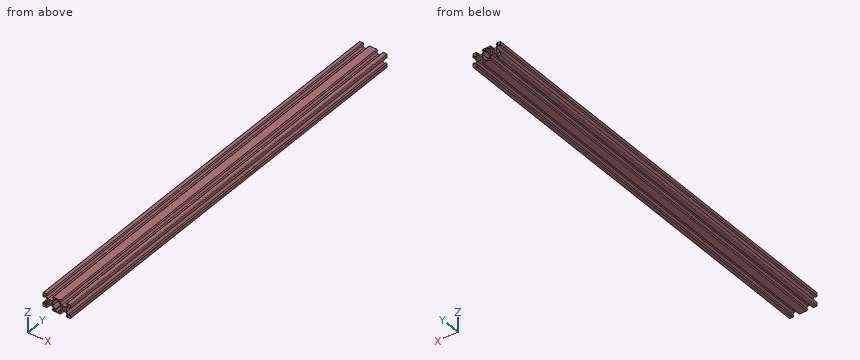
Autodesk Inventor part; units mm, degrees
ref_plane "YZ Plane" through (0, 0, 0) normal (1, 0, 0) x (0, 1, 0)
ref_plane "XZ Plane" through (0, 0, 0) normal (0, 1, 0) x (-1, 0, 0)
ref_plane "XY Plane" through (0, 0, 0) normal (0, 0, 1) x (1, 0, 0)
sketch "Sketch1" plane through (0, 0, 0) normal (0, 1, 0) x (-1, 0, 0)
  line L0 (3.9, -2.8393) -> (3.9, 2.8393)
  line L1 (2.8393, 3.9) -> (-2.8393, 3.9)
  line L2 (-2.8393, -3.9) -> (2.8393, -3.9)
  line L3 (8.5707, 3.2957) -> (10, 4.725)
  line L4 (8.5707, -3.2957) -> (10, -4.725)
  line L5 (8.4, 3.3664) -> (8.4, 6)
  line L6 (8.4, 6) -> (7.0607, 6)
  line L7 (10, 9) -> (10, 4.725)
  line L8 (10, -4.725) -> (10, -9)
  line L9 (3.9, 2.8393) -> (7.0607, 6)
  line L10 (3.2957, 8.5707) -> (4.725, 10)
  line L11 (3.3664, 8.4) -> (6, 8.4)
  line L12 (6, 8.4) -> (6, 7.0607)
  line L13 (2.8393, 3.9) -> (6, 7.0607)
  line L14 (8.4, -3.3664) -> (8.4, -6)
  line L15 (8.4, -6) -> (7.0607, -6)
  line L16 (3.9, -2.8393) -> (7.0607, -6)
  line L17 (3.2957, -8.5707) -> (4.725, -10)
  line L18 (3.3664, -8.4) -> (6, -8.4)
  line L19 (6, -8.4) -> (6, -7.0607)
  line L20 (2.8393, -3.9) -> (6, -7.0607)
  line L21 (-3.9, -2.8393) -> (-3.9, 2.8393)
  line L22 (-3.9, 2.8393) -> (-7.0607, 6)
  line L23 (-6, 8.4) -> (-6, 7.0607)
  line L24 (-2.8393, 3.9) -> (-6, 7.0607)
  line L25 (-3.9, -2.8393) -> (-7.0607, -6)
  line L26 (-2.8393, -3.9) -> (-6, -7.0607)
  line L27 (-6, -8.4) -> (-6, -7.0607)
  line L28 (-3.3664, -8.4) -> (-6, -8.4)
  line L29 (-3.2957, -8.5707) -> (-4.725, -10)
  line L30 (4.725, 10) -> (9, 10)
  line L31 (9, -10) -> (4.725, -10)
  circle A0 centre (0, 0) radius 2.1
  arc A1 (10, 9) -> (9, 10) centre (9, 9) ccw
  arc A2 (9, -10) -> (10, -9) centre (9, -9) ccw
  arc A3 (8.4, 3.3664) -> (8.5707, 3.2957) centre (8.5, 3.3664) ccw
  arc A4 (3.2957, 8.5707) -> (3.3664, 8.4) centre (3.3664, 8.5) ccw
  arc A5 (8.5707, -3.2957) -> (8.4, -3.3664) centre (8.5, -3.3664) ccw
  arc A6 (3.3664, -8.4) -> (3.2957, -8.5707) centre (3.3664, -8.5) ccw
  arc A7 (-3.2957, -8.5707) -> (-3.3664, -8.4) centre (-3.3664, -8.5) ccw
  line L32 (-23.9, -2.8393) -> (-23.9, 2.8393)
  line L33 (-22.8393, 3.9) -> (-17.1607, 3.9)
  line L34 (-17.1607, -3.9) -> (-22.8393, -3.9)
  line L35 (-28.5707, 3.2957) -> (-30, 4.725)
  line L36 (-28.5707, -3.2957) -> (-30, -4.725)
  line L37 (-28.4, 3.3664) -> (-28.4, 6)
  line L38 (-28.4, 6) -> (-27.0607, 6)
  line L39 (-30, 9) -> (-30, 4.725)
  line L40 (-30, -4.725) -> (-30, -9)
  line L41 (-23.9, 2.8393) -> (-27.0607, 6)
  line L42 (-23.2957, 8.5707) -> (-24.725, 10)
  line L43 (-23.3664, 8.4) -> (-26, 8.4)
  line L44 (-26, 8.4) -> (-26, 7.0607)
  line L45 (-22.8393, 3.9) -> (-26, 7.0607)
  line L46 (-23.9, 0) -> (-28.4, 0)
  line L47 (-23.9, -2.8393) -> (-27.0607, -6)
  line L48 (-28.4, -6) -> (-27.0607, -6)
  line L49 (-28.4, -3.3664) -> (-28.4, -6)
  line L50 (-22.8393, -3.9) -> (-26, -7.0607)
  line L51 (-26, -8.4) -> (-26, -7.0607)
  line L52 (-23.3664, -8.4) -> (-26, -8.4)
  line L53 (-23.2957, -8.5707) -> (-24.725, -10)
  line L54 (-16.1, -2.8393) -> (-12.9393, -6)
  line L55 (-17.1607, -3.9) -> (-14, -7.0607)
  line L56 (-16.6336, -8.4) -> (-14, -8.4)
  line L57 (-16.1, -2.8393) -> (-16.1, 2.8393)
  line L58 (-16.1, 2.8393) -> (-12.9393, 6)
  line L59 (-17.1607, 3.9) -> (-14, 7.0607)
  line L60 (-14, 8.4) -> (-14, 7.0607)
  line L61 (-14, -8.4) -> (-14, -7.0607)
  line L62 (-16.7043, -8.5707) -> (-15.275, -10)
  line L63 (-24.725, 10) -> (-29, 10)
  line L64 (-29, -10) -> (-24.725, -10)
  circle A8 centre (-20, 0) radius 2.1
  arc A9 (-29, 10) -> (-30, 9) centre (-29, 9) ccw
  arc A10 (-30, -9) -> (-29, -10) centre (-29, -9) ccw
  arc A11 (-28.5707, 3.2957) -> (-28.4, 3.3664) centre (-28.5, 3.3664) ccw
  arc A12 (-23.3664, 8.4) -> (-23.2957, 8.5707) centre (-23.3664, 8.5) ccw
  arc A13 (-28.4, -3.3664) -> (-28.5707, -3.2957) centre (-28.5, -3.3664) ccw
  arc A14 (-23.2957, -8.5707) -> (-23.3664, -8.4) centre (-23.3664, -8.5) ccw
  arc A15 (-16.6336, -8.4) -> (-16.7043, -8.5707) centre (-16.6336, -8.5) ccw
  arc A16 (-16.7043, 8.5707) -> (-16.6336, 8.4) centre (-16.6336, 8.5) ccw
  line L65 (-7.5, -8.4) -> (-7.5, -6.4393)
  line L66 (-7.0607, -6) -> (-7.5, -6.4393)
  line L67 (-12.5, -7.0607) -> (-12.5, -8.4)
  line L68 (-12.9393, -6) -> (-12.5, -6.4393)
  line L69 (-12.5, -6.4393) -> (-12.5, -7.0607)
  line L70 (-7.5, -8.4) -> (-12.5, -8.4)
  line L71 (-4.725, -10) -> (-15.275, -10)
  line L72 (-3.9, 2.8393) -> (-7.0607, 6)
  line L73 (-2.8393, 3.9) -> (-6, 7.0607)
  line L74 (-3.3664, 8.4) -> (-6, 8.4)
  line L75 (-6, 8.4) -> (-6, 7.0607)
  line L76 (-3.2957, 8.5707) -> (-4.725, 10)
  arc A17 (-3.3664, 8.4) -> (-3.2957, 8.5707) centre (-3.3664, 8.5) ccw
  line L77 (-16.1, 2.8393) -> (-12.9393, 6)
  line L78 (-17.1607, 3.9) -> (-14, 7.0607)
  line L79 (-16.6336, 8.4) -> (-14, 8.4)
  line L80 (-14, 8.4) -> (-14, 7.0607)
  line L81 (-16.7043, 8.5707) -> (-15.275, 10)
  arc A18 (-16.7043, 8.5707) -> (-16.6336, 8.4) centre (-16.6336, 8.5) ccw
  line L82 (-7.5, 8.4) -> (-7.5, 6.4393)
  line L83 (-7.0607, 6) -> (-7.5, 6.4393)
  line L84 (-12.5, 7.0607) -> (-12.5, 8.4)
  line L85 (-12.9393, 6) -> (-12.5, 6.4393)
  line L86 (-12.5, 6.4393) -> (-12.5, 7.0607)
  line L87 (-7.5, 8.4) -> (-12.5, 8.4)
  line L88 (-4.725, 10) -> (-15.275, 10)
extrude "Extrusion1" add sketch "Sketch1" along normal blind 600
properties part number "VSLOT20x40x600"
Geometry check sheet. Reference: the model listing, model coordinates, mm. Coordinates: 2 decimals unless noted, no trailing zeros. Answer as a JSON object with one key per item and string values.
Q1. Cross-section at A-A on y = 355.5. Give the number of separate pieces and of enclosed holes in the cut face, and give its area (3 significant figures).
Results are:
{"separate pieces": "1", "enclosed holes": "3", "area": "281 mm²"}
Q2. Depth check by flat-ended pin: pin 1 Ø1 at (x, y) = (1, 385.5) entering from +Z; pin 2 Ø0.8 at (y, z) = (439, 4.5) entering from +X; pin 3 Ø3 at (y, z) = (296.5, 0) entering from -X; pin 4 Ø6 at (y, z) = (167, -1) entering from +X (3 decimals). Enter the tip coordinate at first touch or a pass-through.
Results are:
{"pin 1": "stops at z = 3.9", "pin 2": "stops at x = 30", "pin 3": "stops at x = -3.9", "pin 4": "stops at x = 29.275"}
Q3. Scan lines: line 1 (Z direction, x = 20.5, y = 326); line 2 (Z direction, x = 0, y = 357); line 3 (Z direction, x = 5.5, y = 299.5). Record each from-to range of solid material in increasing order.
Results are:
{"line 1": "z = -3.9 to -2.04, 2.04 to 3.9", "line 2": "z = -3.9 to -2.1, 2.1 to 3.9", "line 3": "z = -10 to -8.4, -6.56 to -4.44, 4.44 to 6.56, 8.4 to 10"}
